Build history of the part. All positions in model axes, mm. A direction names the side the tool comes from. Round coordinates to 2 decimals unless told otherwise and drop trailing zeros. Order: outer loops, then holes, each group sorted by start corner. A loop starts at its lowest first (then second) coordinate and runs counter-clockwise, first axis right, second up. Notation, with made-up numbers: (-19, 27.25) -> (12, 27.25) arc R15 cw to (12, 49.25) -> close; hole circle Ø4 at (-33, 58). An arc over 180 degrees is marked (long way). Write item = value, one per line.
Autodesk Inventor part; units mm, degrees
ref_plane "YZ Plane" through (0, 0, 0) normal (1, 0, 0) x (0, 1, 0)
ref_plane "XZ Plane" through (0, 0, 0) normal (0, 1, 0) x (-1, 0, 0)
ref_plane "XY Plane" through (0, 0, 0) normal (0, 0, 1) x (1, 0, 0)
sketch "Sketch1" plane through (0, 0, 0) normal (0, 1, 0) x (-1, 0, 0)
  line L0 (12.7, 12.7) -> (-12.7, 12.7)
  line L1 (-12.7, 12.7) -> (-12.7, -12.7)
  line L2 (-12.7, -12.7) -> (12.7, -12.7)
  line L3 (12.7, -12.7) -> (12.7, 12.7)
  line L4 (12.7, 12.7) -> (-12.7, -12.7) construction
  line L5 (-12.7, 12.7) -> (12.7, -12.7) construction
  line L6 (-10.9728, -10.9728) -> (10.9728, -10.9728)
  line L7 (10.9728, -10.9728) -> (10.9728, 10.9728)
  line L8 (10.9728, 10.9728) -> (-10.9728, 10.9728)
  line L9 (-10.9728, 10.9728) -> (-10.9728, -10.9728)
  line L10 (-10.9728, -10.9728) -> (10.9728, 10.9728) construction
  line L11 (10.9728, -10.9728) -> (-10.9728, 10.9728) construction
  point P0 (0, 0)
  dimension "d0" = 25.4
  dimension "d2" = 25.4
  dimension "d3" = 1.7272
extrude "Extrusion1" add sketch "Sketch1" along normal blind 266.7
sketch "Sketch2" plane through (12.7, 0, 12.7) normal (1, 0, 0) x (0, 0, -1)
  line L0 (0, 0) -> (25.4, 0)
  line L1 (25.4, 0) -> (25.4, 266.7)
  line L2 (0, 266.7) -> (25.4, 266.7)
  line L3 (0, 0) -> (0, 266.7)
  point P0 (12.7, 0)
  point P1 (12.7, 254)
  point P2 (12.7, 12.7)
  dimension "d6" = 12.7
  dimension "d7" = 12.7
  dimension "d8" = 12.7
  dimension "d9" = 12.7
hole "Hole1" at (12.7, 254, 0) at (12.7, 12.7, 0) direction (-1, 0, 0) diameter 6.35 end through all
properties part number "CrossBar" material "Aluminum 6061"
Q1. Which spindle directions (+Z, -Z, +X, -X, +Y, -Y) get a long thin tool onto all of the face, cutting with end or side? Do faces 1 (the face through (0.2, 0, 11.5)), 2 (the face through (0, 131, -10.973)). Say none if no direction does.
Check values:
face_1 = +Z, -Z, +X, -X, -Y
face_2 = +Y, -Y
Q2. Mould opens along Y. For faces 3 (the face through (0.2, 266.7, 11.5)), 4 (the face through (11.82, 257.1, 0.69)), 5 (the face through (10.973, 131, 0)) say: released by +Y, released by -Y, zero draft, split by the parting line, or undercut.
Check values:
face_3 = released by +Y
face_4 = undercut
face_5 = zero draft
Q3. Cut at A-A, the plane z = -8.25. List the corners of the cut face in (x, y).
Check values:
outline = (-12.7, 0) -> (-10.97, 0) -> (-10.97, 266.7) -> (-12.7, 266.7) -> close; (10.97, 0) -> (12.7, 0) -> (12.7, 266.7) -> (10.97, 266.7) -> close
Q4. Flat gauge pin, fed straight in: pin 1 (5.5 mm diameter, centred on y = 12.7, z = 0, fed in from +X). Where does the tip first touch, or does it go through?
Check values:
pin_1 = through
Q5. Cut at D-D, the plane y = 106. List the corners of the cut face in (x, z).
Check values:
outline = (-12.7, -12.7) -> (12.7, -12.7) -> (12.7, 12.7) -> (-12.7, 12.7) -> close; hole (-10.97, -10.97) -> (10.97, -10.97) -> (10.97, 10.97) -> (-10.97, 10.97) -> close
Q6. Cut at C-C, the plane y = 12.7. List the corners of the cut face in (x, z) (3 decimals), and give its area (3 significant figures).
Check values:
outline = (-12.7, -12.7) -> (12.7, -12.7) -> (12.7, -3.175) -> (10.973, -3.175) -> (10.973, -10.973) -> (-10.973, -10.973) -> (-10.973, -3.175) -> (-12.7, -3.175) -> close; (-12.7, 3.175) -> (-10.973, 3.175) -> (-10.973, 10.973) -> (10.973, 10.973) -> (10.973, 3.175) -> (12.7, 3.175) -> (12.7, 12.7) -> (-12.7, 12.7) -> close
area = 142 mm²
Q7. Cut at B-B, the plane x = -4. List the corners of the cut face in (y, z), and give its area (3 significant figures).
Check values:
outline = (0, -12.7) -> (266.7, -12.7) -> (266.7, -10.97) -> (0, -10.97) -> close; (0, 10.97) -> (266.7, 10.97) -> (266.7, 12.7) -> (0, 12.7) -> close
area = 921 mm²
Q8. Probe probe 1 along Y at (x, z) = (-11.65, 0) (3 decimals); probe 2 along Z at (x, y) = (1, 101). List the from-to ranges inside material, lowest first.
Check values:
probe_1 = 0 to 9.525, 15.875 to 250.825, 257.175 to 266.7
probe_2 = -12.7 to -10.97, 10.97 to 12.7
